Verification items for the finished model (mm, model axes). Give positions to 0.01 mm unless a question says otherwise; leave off trailing zeros. Loops run counter-clockwise (first coordinate to the right, second up) from the corner with the lowest first, then second, coordinate; pieces in that order, holes last. Notation, with made-up numbers: (84, 89.5) - (88, 89.5) arc R29 cw to (88, 122.5) - close; hole circle Ø3 at (-28, 25). An arc over 180 degrees is marked (long way). Answer in a Markdown table with one row per item.
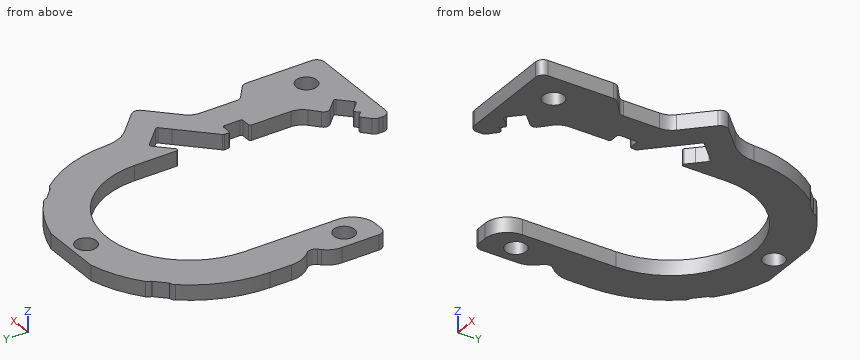
```python
from build123d import *

# Parameters (mm, degrees)
CORPS_DEPTH                     = 4
DIAM_TRE_DU_PER_AGE_5_5_5_5_2_D = 5.5
RENFORT_CAVITE_IR_DEPTH         = 4
CAVITE_IR_DEPTH                 = 73.870494144
CAVITE_SWITCH_DEPTH             = 73.870494144
CONG_1_R                        = 2
CONG_1_R_2                      = 5
CONG_1_R_3                      = 10
CONG_1_R_4                      = 8
CONG_1_R_5                      = 6
CONG_1_R_6                      = 1.5
CONG_2_R                        = 0.5


with BuildPart() as part:
    # Esquisse1 → corps (new body)
    with BuildSketch(Plane.XY):
        with BuildLine():
            Line((-21.1677086, 23.996135725), (-21.1677086, 24.661267457))
            ThreePointArc((-21.1677086, 24.661267457), (-14.979348182, 28.84214153), (-8, 31.5))
            Line((-8, 31.5), (8, 31.5))
            ThreePointArc((8, 31.5), (14.979348182, 28.84214153), (21.1677086, 24.661267457))
            Line((21.1677086, 24.661267457), (21.1677086, 23.996135725))
            Line((21.1677086, 23.996135725), (23.996135725, 21.1677086))
            Line((23.996135725, 21.1677086), (24.661267457, 21.1677086))
            ThreePointArc((24.661267457, 21.1677086), (30.477378434, 11.286248439), (32.5, 0))
            Line((32.5, 0), (32.5, -35))
            Line((32.5, -35), (37.5, -39))
            Line((37.5, -39), (37.5, -59.4))
            Line((37.5, -59.4), (8.886620253, -59.4))
            Line((8.886620253, -59.4), (8.886620253, -56.358407696))
            ThreePointArc((8.886620253, -56.358407696), (9.059529338, -55.54493441), (9.54835904, -54.872118045))
            Line((9.54835904, -54.872118045), (20.413163329, -45.089404323))
            ThreePointArc((20.413163329, -45.089404323), (21.585367396, -43.476003838), (22, -41.525310806))
            Line((22, -41.525310806), (22, 0))
            ThreePointArc((22, 0), (0, 22), (-22, 0))
            Line((-22, 0), (-22, -24.928632557))
            ThreePointArc((-22, -24.928632557), (-23.757359313, -29.171273244), (-28, -30.928632557))
            Line((-28, -30.928632557), (-32.5, -30.928632557))
            Line((-32.5, -30.928632557), (-32.5, 0))
            ThreePointArc((-32.5, 0), (-30.477378434, 11.286248439), (-24.661267457, 21.1677086))
            Line((-24.661267457, 21.1677086), (-23.996135725, 21.1677086))
            Line((-23.996135725, 21.1677086), (-21.1677086, 23.996135725))
        make_face()
    extrude(amount=CORPS_DEPTH)

    # Diamètre du perçage Ø5.5 (5.5)2 (through all)
    with Locations(Plane.XY.offset(4)):
        with Locations((0, 27.5), (30, -51), (-27.5, -23)):
            Hole(DIAM_TRE_DU_PER_AGE_5_5_5_5_2_D / 2)

    # Esquisse4 → renfort_cavite_IR (add, through all)
    with BuildSketch(Plane.XY):
        Polygon((31.767766953, -2.575378798), (42.02081528, -12.828427125), (34.87903679, -19.970205615), (27.454415588, -27.394826817), (24.625988463, -9.717157288), align=None)
    extrude(amount=RENFORT_CAVITE_IR_DEPTH)

    # Esquisse4<4> → cavite_IR (cut, through all)
    with BuildSketch(Plane.XY):
        Polygon((0, -34.343145751), (24.625988463, -9.717157288), (27.171572875, -7.171572875), (32.828427125, -12.828427125), (30.282842712, -15.374011537), (0, -45.656854249), align=None)
        Polygon((-75.939696962, -31.797561338), (-42.828427125, 1.313708499), (-28.686291501, -12.828427125), (-61.797561338, -45.939696962), align=None)
    extrude(amount=CAVITE_IR_DEPTH, mode=Mode.SUBTRACT)

    # Esquisse5 → cavite_switch (cut, through all)
    with BuildSketch(Plane.XY):
        Polygon((13.884745674, -52.561700936), (12.661450942, -51.338406204), (16.338406204, -47.661450942), (17.561700936, -48.884745674), (17.915254326, -49.238299064), (20.920458146, -52.243502884), (20.991168825, -52.314213562), (17.314213562, -55.991168825), (17.243502884, -55.920458146), (14.238299064, -52.915254326), align=None)
        Polygon((13.884745674, -52.561700936), (12.661450942, -51.338406204), (11.459369414, -52.540487732), (13.177638892, -54.258757211), (14.37972042, -53.056675683), (14.238299064, -52.915254326), align=None)
        Polygon((18.52, -25.4), (20.25, -25.4), (20.75, -25.4), (25, -25.4), (25.1, -25.4), (25.1, -30.6), (25, -30.6), (20.75, -30.6), (20.25, -30.6), (18.52, -30.6), align=None)
        Polygon((20.75, -30.6), (20.25, -30.6), (18.52, -30.6), (18.52, -32.3), (20.95, -32.3), (20.95, -30.6), align=None)
    extrude(amount=CAVITE_SWITCH_DEPTH, mode=Mode.SUBTRACT)

    # Congé1
    # the kernel refuses this fillet: 10, 8, 6, 5, 2, 1.5 mm, written as the material it adds along each edge
    with BuildSketch(Plane(origin=(-28.686291501, -12.828427125, 0), x_dir=(-0.7071067811865516, 0.7071067811865436, 0), z_dir=(0, 0, 1))) as cong_1_piece_1:
        with BuildLine():
            CenterArc((CONG_1_R, CONG_1_R), CONG_1_R, 180, 90)
            Line((0, CONG_1_R), (0, 0))
            Line((0, 0), (CONG_1_R, 0))
        make_face()
    extrude(amount=4)
    with BuildSketch(Plane(origin=(32.5, -35, 0), x_dir=(0.7808688094430325, -0.6246950475544215, 0), z_dir=(0, 0, 1))) as cong_1_piece_2:
        with BuildLine():
            CenterArc((CONG_1_R * 0.480624847487, CONG_1_R), CONG_1_R, 218.659808254, 51.340191746)
            Line((-CONG_1_R * 0.300243961956, CONG_1_R * 0.375304952446), (0, 0))
            Line((0, 0), (CONG_1_R * 0.480624847487, 0))
        make_face()
    extrude(amount=4)
    with BuildSketch(Plane(origin=(32.5, -22.349242405, 4), x_dir=(0, -1, 0), z_dir=(0, 0, -1))) as cong_1_piece_3:
        with BuildLine():
            CenterArc((CONG_1_R_2 * 0.414213562373, -CONG_1_R_2), CONG_1_R_2, 90, 45)
            Line((-CONG_1_R_2 * 0.292893218813, -CONG_1_R_2 * 0.292893218813), (0, 0))
            Line((0, 0), (CONG_1_R_2 * 0.414213562373, 0))
        make_face()
    extrude(amount=4)
    with BuildSketch(Plane(origin=(32.5, -3.307611845, 0), x_dir=(0.7071067811865513, -0.7071067811865438, 0), z_dir=(0, 0, 1))) as cong_1_piece_4:
        with BuildLine():
            CenterArc((4.130314106, 10), CONG_1_R_3, 226.136395215, 43.863604785)
            Line((-2.799125719, 2.790085736), (-3.492069702, 2.069094309))
            ThreePointArc((-3.492069702, 2.069094309), (-3.045941546, 1.631727984), (-0.707106781, -0.707106781))
            Line((-0.707106781, -0.707106781), (0, -1))
            Line((0, -1), (4.130314106, -1))
            Line((4.130314106, -1), (4.130314106, 0))
        make_face()
    extrude(amount=4)
    # the kernel refuses this fillet: 10, 8, 6, 5, 2, 1.5 mm, written as the material it takes off along each edge
    with BuildSketch(Plane(origin=(-32.5, -30.928632557, -5), x_dir=(0, 1, 0), z_dir=(0, 0, 1)), Plane(origin=(37.5, -59.4, -5), x_dir=(-1, 0, 0), z_dir=(0, 0, 1)), Plane(origin=(42.02081528, -12.828427125, -5), x_dir=(-0.7071067811865427, -0.7071067811865525, 0), z_dir=(0, 0, 1)), Plane(origin=(8.886620253, -59.4, -5), x_dir=(0, 1, 0), z_dir=(0, 0, 1))) as cong_1_2_piece_1:
        with BuildLine():
            CenterArc((CONG_1_R, -CONG_1_R), CONG_1_R, 90, 90)
            Line((0, -CONG_1_R), (0, 0))
            Line((0, 0), (CONG_1_R, 0))
        make_face()
    extrude(amount=14, mode=Mode.SUBTRACT)
    with BuildSketch(Plane(origin=(37.5, -39, -2.403124237), x_dir=(0, -1, 0), z_dir=(0, 0, 1))) as cong_1_2_piece_2:
        with BuildLine():
            CenterArc((CONG_1_R * 0.480624847487, -CONG_1_R), CONG_1_R, 90, 51.340191746)
            Line((-CONG_1_R * 0.300243961956, -CONG_1_R * 0.375304952446), (0, 0))
            Line((0, 0), (CONG_1_R * 0.480624847487, 0))
        make_face()
    extrude(amount=8.806248475, mode=Mode.SUBTRACT)
    with BuildSketch(Plane(origin=(21.1677086, 24.661267457, -2.345925687), x_dir=(0, -1, 0), z_dir=(0, 0, 1)), Plane(origin=(-24.661267457, 21.1677086, -2.345925687), x_dir=(1, 0, 0), z_dir=(0, 0, 1))) as cong_1_2_piece_3:
        with BuildLine():
            CenterArc((0.953759933, -1.97906386), CONG_1_R, 98.297562286, 42.71603868)
            ThreePointArc((-0.600830724, -0.720792074), (-0.30301692, -0.358227456), (0, 0))
            Line((0, 0), (0.665131732, 0))
        make_face()
    extrude(amount=8.691851375, mode=Mode.SUBTRACT)
    with BuildSketch(Plane(origin=(24.661267457, 21.1677086, -2.345925687), x_dir=(-1, 0, 0), z_dir=(0, 0, 1)), Plane(origin=(-21.1677086, 24.661267457, -2.345925687), x_dir=(0, -1, 0), z_dir=(0, 0, 1))) as cong_1_2_piece_4:
        with BuildLine():
            CenterArc((0.953759933, 1.97906386), CONG_1_R, 218.986399033, 42.71603868)
            ThreePointArc((-0.600830724, 0.720792074), (-0.30301692, 0.358227456), (0, 0))
            Line((0, 0), (0.665131732, 0))
        make_face()
    extrude(amount=8.691851375, mode=Mode.SUBTRACT)
    with BuildSketch(Plane(origin=(-32.5, -9.014718626, 12.284271247), x_dir=(0, 1, 0), z_dir=(0, 0, -1))) as cong_1_2_piece_5:
        with BuildLine():
            CenterArc((CONG_1_R_4 * 0.414213562373, CONG_1_R_4), CONG_1_R_4, 225, 45)
            Line((-CONG_1_R_4 * 0.292893218813, CONG_1_R_4 * 0.292893218813), (0, 0))
            Line((0, 0), (CONG_1_R_4 * 0.414213562373, 0))
        make_face()
    extrude(amount=20.568542495, mode=Mode.SUBTRACT)
    with BuildSketch(Plane(origin=(-32.5, -16.642135624, -6.213203436), x_dir=(0.7071067811865432, 0.7071067811865519, 0), z_dir=(0, 0, 1))) as cong_1_2_piece_6:
        with BuildLine():
            CenterArc((CONG_1_R_5 * 0.414213562373, -CONG_1_R_5), CONG_1_R_5, 90, 45)
            Line((-CONG_1_R_5 * 0.292893218813, -CONG_1_R_5 * 0.292893218813), (0, 0))
            Line((0, 0), (CONG_1_R_5 * 0.414213562373, 0))
        make_face()
    extrude(amount=16.426406871, mode=Mode.SUBTRACT)
    with BuildSketch(Plane(origin=(16.915589345, -48.238634083, 7.95167547), x_dir=(0.7431448254773909, 0.6691306063588618, 0), z_dir=(0, 0, -1))) as cong_1_2_piece_7:
        with BuildLine():
            CenterArc((CONG_1_R_6 * 1.05378012528, CONG_1_R_6), CONG_1_R_6, 177, 93)
            Line((CONG_1_R_6 * 0.0551505905264, CONG_1_R_6 * 1.05233595624), (0, 0))
            Line((0, 0), (CONG_1_R_6 * 1.05378012528, 0))
        make_face()
    extrude(amount=11.90335094, mode=Mode.SUBTRACT)

    # Congé2
    cong_2_edges = [part.edges().sort_by_distance(p)[0] for p in [
        (22, -12.343145751, 2),
        (27.171572875, -7.171572875, 2),
        (22, -23.656854249, 2),
        (32.828427125, -12.828427125, 2),
        (11.780853072, -52.86197139, 2),
        (20.991168825, -52.314213562, 2),
        (14.37972042, -53.056675683, 2),
        (17.314213562, -55.991168825, 2),
        (22, -25.4, 2),
        (25.1, -25.4, 2),
        (22, -30.6, 2),
        (25.1, -30.6, 2),
    ]]
    fillet(cong_2_edges, radius=CONG_2_R)


solid = part.part
```
Q1. Sectioned sample at A-A (x = 0). Record the cut outline in (y, z), and give its area (3 significant figures).
Completed:
| item | result |
|---|---|
| outline | (22, 0) - (24.75, 0) - (24.75, 4) - (22, 4) - close; (30.25, 0) - (31.5, 0) - (31.5, 4) - (30.25, 4) - close |
| area | 16.0 mm^2 |
Q2. Thickness scan on line 1 (Y direction, x = 0, z = 2.8); line 2 (Y direction, x = 30, z = 3.05); line 3 (Y direction, x = 22.5, z = 2.2). Record the ranges inside material, lowest first.
Completed:
| item | result |
|---|---|
| line 1 | 22 to 24.75, 30.25 to 31.5 |
| line 2 | -59.4 to -53.75, -48.25 to -15.66, -10 to 12.5 |
| line 3 | -59.4 to -30.6, -25.4 to -23.16, -11.64 to 22.66 |
Q3. Sectioned sample at C-C (y = -22). Record the cut outline in (x, z), and give its area (3 significant figures).
Completed:
| item | result |
|---|---|
| outline | (-32.5, 0) - (-30.06, 0) - (-30.06, 4) - (-32.5, 4) - close; (-24.94, 0) - (-22, 0) - (-22, 4) - (-24.94, 4) - close; (23.66, 0) - (33.12, 0) - (33.12, 4) - (23.66, 4) - close |
| area | 59.4 mm^2 |
Q4. Go/stop test with flat-tipped pins: P1, Ø2, axis at y = -47.5, z = 1.5, coming from the +X side; P2, Ø2, axis at y = -18.5, z = 2, coming from the +X side; P3, Ø1.2, axis at y = -35.5, z = 1, coming from the -X side. Record where each tip stops, or that it passes through.
Completed:
| item | result |
|---|---|
| P1 | x = 37.5 |
| P2 | x = 37.35 |
| P3 | x = 22 |
Q5. Sectioned sample at B-B (y = -4). Record the cut outline in (x, z), and give its area (3 significant figures).
Completed:
| item | result |
|---|---|
| outline | (-32.5, 0) - (-22, 0) - (-22, 4) - (-32.5, 4) - close; (22, 0) - (33.74, 0) - (33.74, 4) - (22, 4) - close |
| area | 89.0 mm^2 |
Q6. Sectioned sample at D-D (z = 3.25). Give the number of separate pieces and of enclosed holes in the cut face, and give its area (3 significant figures).
Completed:
| item | result |
|---|---|
| separate pieces | 1 |
| enclosed holes | 3 |
| area | 1,930 mm^2 |
